from build123d import *

# Parameters (mm, degrees)
SKETCH1_R           = 20.555
SKETCH1_R_2         = 19.305
BOSS_EXTRUDE3_DEPTH = 400
SKETCH2_W           = 3.5
SKETCH2_H           = 46
CUT_EXTRUDE1_DEPTH  = 21.555
CIRPATTERN1_COUNT   = 2
CIRPATTERN1_ANGLE   = 90


with BuildPart() as part:
    # Sketch1 → Boss-Extrude3 (new body)
    with BuildSketch(Plane.XY):
        Circle(SKETCH1_R)
        Circle(SKETCH1_R_2, mode=Mode.SUBTRACT)
    extrude(amount=-BOSS_EXTRUDE3_DEPTH)

    # Sketch2 → Cut-Extrude1 (cut, symmetric)
    with BuildSketch(Plane(origin=(0, 0, 0), x_dir=(1, 0, 0), z_dir=(0, 1, 0))):
        with Locations((0, 34)):
            Rectangle(SKETCH2_W, SKETCH2_H)
    cut_extrude1 = extrude(amount=CUT_EXTRUDE1_DEPTH, both=True, mode=Mode.SUBTRACT)

    # CirPattern1: Cut-Extrude1 ×2 about axis
    cirpattern1_axis = Axis((0, 0, -400), (0, 0, 1))
    for i in range(1, CIRPATTERN1_COUNT):
        add(cut_extrude1.rotate(cirpattern1_axis, i * CIRPATTERN1_ANGLE / (CIRPATTERN1_COUNT - 1)), mode=Mode.SUBTRACT)


solid = part.part
The listing builds one solid part. Answer for the finished solid, in the listing's coordinates (mm). Give positions to 0.01 mm unless a question says otherwise; leave off trailing zeros. Order: outer loops, then holes, each group sorted by start corner. A loop starts at its lowest first (then second) coordinate and runs counter-clockwise, first axis right, second up. Notation, with made-up numbers: (42.25, 75.25) -> (49.25, 75.25) arc R26 ccw to (49.25, 90.25) -> close; hole circle Ø9 at (82, -24). An arc over 180 degrees is marked (long way). Put each result on its own line as item: value.
Item 1: For a pull along X with two mould halves and no side action, classify faces 1 (the face through (19.606, 6.174, -197.2)), 2 (the face through (18.414, 5.799, -197.2)) as released by +X, released by -X, zero draft, split by the parting line, or undercut.
Established:
face 1: split by the parting line
face 2: undercut
Item 2: A cutting plane is placed at B-B on y = -13.5. Give the vertices of the cut face in (x, z).
Established:
outline: (-15.5, -400) -> (-13.8, -400) -> (-13.8, 0) -> (-15.5, 0) -> close; (13.8, -400) -> (15.5, -400) -> (15.5, 0) -> (13.8, 0) -> close
Item 3: A cutting plane is placed at A-A on x = -7.5. Give the vertices of the cut face in (y, z), plus the area to 3 significant figures.
Established:
outline: (-19.14, -400) -> (-17.79, -400) -> (-17.79, 0) -> (-19.14, 0) -> close; (17.79, -400) -> (19.14, -400) -> (19.14, 0) -> (17.79, 0) -> close
area: 1,080 mm^2
Item 4: Given P1, Ø0.7, axis at x = 20, y = -0.5, coming from the +Z side; P2, Ø10, axis at x = -9.5, z = -173, coming from the +Y side; P3, Ø8, axis at x = -13, z = -311.5, coming from the -Y side; P4, Ø2, axis at y = 16, z = -145.5, coming from the +X side, each flat-ended and moving along its own axis, determine where each tip first touches the part or whether it passes through.
Established:
P1: stops at z = 0
P2: stops at y = 20.06
P3: stops at y = -18.48
P4: stops at x = 14.05
Item 5: Straight lines are drawn through the part: line 1 (Y direction, x = 0, z = -115) (3 decimals); line 2 (Y direction, x = -2, z = -57). For each, find the intervals that lie inside material, in ascending order.
Established:
line 1: y = -20.555 to -19.305, 19.305 to 20.555
line 2: y = -20.46 to -19.2, 19.2 to 20.46
Item 6: A cutting plane is placed at C-C on z = -158. Give the vertices of the cut face in (x, y) (3 decimals).
Established:
outline: circle Ø41.11 at (0, 0); hole circle Ø38.61 at (0, 0)
